Autodesk Inventor part; units mm, degrees
ref_plane "YZ Plane" through (0, 0, 0) normal (1, 0, 0) x (0, 1, 0)
ref_plane "XZ Plane" through (0, 0, 0) normal (0, 1, 0) x (-1, 0, 0)
ref_plane "XY Plane" through (0, 0, 0) normal (0, 0, 1) x (1, 0, 0)
sketch "Sketch1" plane through (0, 0, 0) normal (0, 0, 1) x (1, 0, 0)
  line L0 (0, 33) -> (0, -1)
  line L1 (0, -1) -> (3.75, -1) construction
  line L2 (3.75, -1) -> (3.75, 0)
  line L3 (3.75, 0) -> (10, 0)
  line L4 (10, 0) -> (10, 20)
  line L5 (10, 20) -> (8, 20)
  line L6 (8, 20) -> (8, 24)
  line L7 (8, 24) -> (6, 24)
  line L8 (6, 24) -> (6, 25)
  line L9 (6, 25) -> (5, 25)
  line L10 (5, 25) -> (5, 27)
  line L11 (5, 27) -> (6, 27)
  line L12 (6, 27) -> (6, 33)
  line L13 (6, 33) -> (0, 33)
  line L14 (10, 0) -> (0, 0) construction
  line L15 (6, 24) -> (6, 33) construction
  line L16 (2.5, 33) -> (2.5, 19)
  line L17 (2.5, 19) -> (1.55, 19)
  line L18 (1.55, 19) -> (1.55, 17)
  line L19 (1.55, 17) -> (2, 17)
  line L20 (10, 19.1818) -> (4.75, 19.1818)
  line L21 (4.75, 19.1818) -> (4.75, 18.0818)
  line L22 (4.75, 18.0818) -> (10, 18.0818)
  line L23 (10, 17.2636) -> (4.75, 17.2636)
  line L24 (4.75, 16.1636) -> (4.75, 17.2636)
  line L25 (4.75, 16.1636) -> (10, 16.1636)
  line L26 (10, 15.3455) -> (4.75, 15.3455)
  line L27 (4.75, 15.3455) -> (4.75, 14.2455)
  line L28 (4.75, 14.2455) -> (10, 14.2455)
  line L29 (10, 13.4273) -> (4.75, 13.4273)
  line L30 (4.75, 13.4273) -> (4.75, 12.3273)
  line L31 (4.75, 12.3273) -> (10, 12.3273)
  line L32 (10, 11.5091) -> (4.75, 11.5091)
  line L33 (4.75, 11.5091) -> (4.75, 10.4091)
  line L34 (4.75, 10.4091) -> (10, 10.4091)
  line L35 (10, 9.5909) -> (4.75, 9.5909)
  line L36 (4.75, 9.5909) -> (4.75, 8.4909)
  line L37 (4.75, 8.4909) -> (10, 8.4909)
  line L38 (10, 7.6727) -> (4.75, 7.6727)
  line L39 (4.75, 7.6727) -> (4.75, 6.5727)
  line L40 (4.75, 6.5727) -> (10, 6.5727)
  line L41 (10, 5.7545) -> (4.75, 5.7545)
  line L42 (4.75, 5.7545) -> (4.75, 4.6545)
  line L43 (4.75, 4.6545) -> (10, 4.6545)
  line L44 (4.75, 18.0818) -> (4.75, 17.2636) construction
  line L45 (4.75, 16.1636) -> (4.75, 15.3455) construction
  line L46 (4.75, 14.2455) -> (4.75, 13.4273) construction
  line L47 (4.75, 12.3273) -> (4.75, 11.5091) construction
  line L48 (4.75, 10.4091) -> (4.75, 9.5909) construction
  line L49 (4.75, 8.4909) -> (4.75, 7.6727) construction
  line L50 (4.75, 6.5727) -> (4.75, 5.7545) construction
  line L51 (10, 3.8364) -> (4.75, 3.8364)
  line L52 (4.75, 3.8364) -> (4.75, 2.7364)
  line L53 (4.75, 2.7364) -> (10, 2.7364)
  line L54 (10, 1.9182) -> (4.75, 1.9182)
  line L55 (4.75, 1.9182) -> (4.75, 0.8182)
  line L56 (4.75, 0.8182) -> (10, 0.8182)
  line L57 (4.75, 4.6545) -> (4.75, 3.8364) construction
  line L58 (4.75, 2.7364) -> (4.75, 1.9182) construction
  line L59 (4.75, 0) -> (4.75, 0.8182) construction
  line L60 (8, 20) -> (8, 19.1818) construction
  line L61 (8, 23) -> (4.75, 23)
  line L62 (4.75, 23) -> (4.75, 21.9)
  line L63 (4.75, 21.9) -> (8, 21.9)
  line L64 (8, 20) -> (4.75, 20)
  line L65 (8, 21.1) -> (4.75, 21.1)
  line L66 (4.75, 21.1) -> (4.75, 20)
  line L67 (3, -1) -> (3, 0)
  line L68 (3.75, -1) -> (3, -1)
  line L69 (2, 17) -> (2, 0)
  line L70 (3, 0) -> (2, 0)
  point P0 (5.5, 25)
  dimension "d2" = 12
  dimension "d3" = 20
  dimension "d4" = 7.5
  dimension "d5" = 20
  dimension "d6" = 16
  dimension "d7" = 10
  dimension "d11" = 6
  dimension "d12" = 8
  dimension "d13" = 33
  dimension "d14" = 5
  dimension "d16" = 3.1
  dimension "d17" = 17
  dimension "d18" = 14
  dimension "d19" = 9
  dimension "d21" = 1.1
  dimension "d25" = 9.5
  dimension "d26" = 1
  dimension "d27" = 0.8
  dimension "d28" = 1
  dimension "d29" = 6
  dimension "d30" = 4
revolve "Revolution1" add sketch "Sketch1" angle 360 about axis through (0, 33, 0) along (0, -1, 0) contours L68 L67 L70 L69 L19 L18 L17 L16 L13 L12 L11 L10 L9 L8 L7 L6 L61 L62 L63 L65 L66 L64 L5 L4 L20 L21 L22 L23 L24 L25 L26 L27 L28 L29 L30 L31 L32 L33 L34 L35 L36 L37 L38 L39 L40 L41 L42 L43 L51 L52 L53 L54 L55 L56 L3 L2
properties part number "REVO-micro Heatsing body" material "Aluminum 6061"
Input: part model. Units: mm. Frame: model coordinates. A direction names the side the tool comes from. Coordinates: 2 decimals unless noted, no trailing zeros. Answer as CSV lines item,"result".
1. Material intervals for line 1 (Z direction, x = 0, y = 11.75); line 2 (Y direction, x = -0.25, z = 4.25); line 3 (Z direction, x = 2.25, y = 32), sorted ascending. Write a range as from..to.
Reported:
line 1,"-10..-2, 2..10"
line 2,"0..33"
line 3,"-5.56..-1.09, 1.09..5.56"
2. Section A-A (x = 6.5). State how many separate pieces and enclosed holes the cut face has, then the cut area to 3 significant figures.
Reported:
separate pieces,"13"
enclosed holes,"0"
area,"154 mm2"
3. Access query for faces 1 (the flat face through (0, 21.1, -5)), 2 (the cylindrical face through (-1.73, 21.51, 7.81)), 3 (the cylindrical face through (-2.17, 15.76, 9.76)), 4 (the cylindrical face through (-3, -0.5, -0.1)). Directions: +Z, -Z, +X, -X, +Y, -Y. A direction counts if a zero-diameter tool reaches every point of the face in a straight line with its end or side. Return the directions, or none.
Reported:
face 1,"none"
face 2,"+Y"
face 3,"+Y, -Y"
face 4,"-Y"
4. Pull-direction query (Y, two-part tool) for faces 5 (the flat face through (-4, 25, 4)), 6 (the cylindrical face through (-2.17, 11.92, 9.76)), 7 (the flat face through (1, -1, 3)); classes: released by +Y, released by -Y, zero draft, split by the parting line, or undercut.
Reported:
face 5,"undercut"
face 6,"zero draft"
face 7,"released by -Y"
5. First-contact query: P1, Ø1, axis at x = 0, z = 0, coming from the +Y side; P2, Ø1, axis at x = 4, z = -3, coming from the -Y side; P3, Ø6, axis at y = 23.5, z = -7, coming from the +X side; P4, Ø8, axis at x = 0.5, y = 27.5, coming from the +Z side. Flat tips, straight axial feed; report the tip coordinate or a pass-through.
Reported:
P1,"through"
P2,"y = 0"
P3,"x = 6.93"
P4,"z = 8"
